```python
from build123d import *

# Parameters (mm, degrees)
SKETCH1_W           = 37.4
SKETCH1_H           = 57.2
BOSS_EXTRUDE1_DEPTH = 12.5
SHELL1_T            = -2
CUT_EXTRUDE1_DEPTH  = 70.475535262
SKETCH3_W           = 33
SKETCH3_H           = 8
BOSS_EXTRUDE2_DEPTH = 15
SKETCH4_W           = 5
SKETCH4_H           = 23
CUT_EXTRUDE2_DEPTH  = 82.955246934
FILLET2_R           = 1


with BuildPart() as part:
    # Sketch1 → Boss-Extrude1 (new body)
    with BuildSketch(Plane(origin=(0, 0, 0), x_dir=(0, 1, 0), z_dir=(0, 0, 1))):
        with Locations((-18.7, 28.6)):
            Rectangle(SKETCH1_W, SKETCH1_H)
    extrude(amount=BOSS_EXTRUDE1_DEPTH)

    # Shell1
    shell1_openings = [part.faces().sort_by_distance(p)[0] for p in [
        (0, -18.7, 6.25),
    ]]
    offset(amount=SHELL1_T, openings=shell1_openings, kind=Kind.INTERSECTION)

    # Sketch2 → Cut-Extrude1 (cut, through all)
    with BuildSketch(Plane.XY.offset(12.5)):
        with BuildLine():
            Line((-51.1, -37.4), (-51.1, -35.4))
            ThreePointArc((-51.1, -35.4), (-48.35, -32.65), (-45.6, -35.4))
            Line((-45.6, -35.4), (-45.6, -37.4))
            Line((-45.6, -37.4), (-51.1, -37.4))
        make_face()
        with BuildLine():
            Line((-51.1, 0), (-51.1, -2))
            ThreePointArc((-51.1, -2), (-48.35, -4.75), (-45.6, -2))
            Line((-45.6, -2), (-45.6, 0))
            Line((-45.6, 0), (-51.1, 0))
        make_face()
    extrude(amount=-CUT_EXTRUDE1_DEPTH, mode=Mode.SUBTRACT)

    # Sketch3 → Boss-Extrude2 (add)
    with BuildSketch(Plane(origin=(-57.2, 0, 0), x_dir=(0, -1, 0), z_dir=(-1, 0, 0))):
        with Locations((18.7, 6.25)):
            Rectangle(SKETCH3_W, SKETCH3_H)
    extrude(amount=BOSS_EXTRUDE2_DEPTH)

    # Sketch4 → Cut-Extrude2 (cut, through all)
    with BuildSketch(Plane(origin=(0, 0, 2.25), x_dir=(1, 0, 0), z_dir=(0, 0, -1))):
        with Locations((-64.7, 18.7)):
            Rectangle(SKETCH4_W, SKETCH4_H)
    extrude(amount=-CUT_EXTRUDE2_DEPTH, mode=Mode.SUBTRACT)

    # Fillet2
    fillet2_edges = [part.edges().sort_by_distance(p)[0] for p in [
        (-54.15, -37.4, 12.5),
        (-53.15, -35.4, 10.5),
        (-54.15, 0, 0),
        (-22.8, -37.4, 0),
        (-54.15, 0, 12.5),
        (-22.8, -37.4, 12.5),
        (-45.6, -37.4, 6.25),
        (-51.1, -37.4, 6.25),
        (-22.8, 0, 12.5),
        (-51.1, 0, 6.25),
        (-45.6, 0, 6.25),
        (-54.15, -37.4, 0),
        (-57.2, -18.7, 0),
        (-22.8, 0, 0),
        (-57.2, -35.2, 6.25),
        (-64.7, -35.2, 2.25),
        (-57.2, -18.7, 10.25),
        (-64.7, -35.2, 10.25),
        (-57.2, -2.2, 6.25),
        (-64.7, -2.2, 10.25),
        (-57.2, -18.7, 2.25),
        (-64.7, -2.2, 2.25),
        (-72.2, -35.2, 6.25),
        (-72.2, -18.7, 10.25),
        (-72.2, -2.2, 6.25),
        (-72.2, -18.7, 2.25),
        (-57.2, -37.4, 6.25),
        (-57.2, 0, 6.25),
        (-64.7, -7.2, 10.25),
        (-62.2, -7.2, 6.25),
        (-67.2, -18.7, 10.25),
        (-67.2, -7.2, 6.25),
        (-64.7, -30.2, 10.25),
        (-67.2, -30.2, 6.25),
        (-62.2, -18.7, 10.25),
        (-62.2, -30.2, 6.25),
        (-64.7, -7.2, 2.25),
        (-62.2, -18.7, 2.25),
        (-57.2, -18.7, 12.5),
        (-64.7, -30.2, 2.25),
        (-67.2, -18.7, 2.25),
    ]]
    fillet(fillet2_edges, radius=FILLET2_R)


solid = part.part
```
Verification items for the finished model (mm, model axes). A direction names the side the tool comes from. Coordinates: 2 decimals unless noted, no trailing zeros. Loops run counter-clockwise (first coordinate to the right, second up) from the corner with the lowest first, then second, coordinate; pieces in that order, holes last. Notation, with made-up numbers: (72.25, 25) -> (105.25, 25) arc R29 ccw to (105.25, 56) -> close; hole circle Ø1 at (-27.75, 5). An arc over 180 degrees is marked (long way). Answer in a Markdown table with one row per item. Add a question column.
1. Section check D-D, the plane z = 8. Give the number of separate pieces and of enclosed holes in the cut face, then the cut area to 3 significant figures.
2. Section check C-C, the plane x = -20. Enter the section's corners in (y, z).
3. Access from +Z, -Z, +X, -X, +Y, -Y to the whole of each face (thin tool, end or side, straight path). Record for faces 4 (the face through (-65, -35.2, 6)), 5 (the face through (-69, -18, 10.25)), 6 (the face through (-53, -2, 6)).
4. Material ranges on probe 1 along X at (y, z) = (-13.5, 8.75); probe 2 along Z at (x, y) = (-44, -35); probe 3 along Y at (x, z) = (-31, 9.25), recorded low to high. Write a range as [from, to].
5. Section check B-B, the plane y = -14. Enter the section's corners in (x, z), then the cut area to 3 significant figures.
6. Section check A-A, the plane x = -65. Enter the section's corners in (y, z).
7. Depth check by flat-ended pin: P1, Ø0.5, axis at y = -1.5, z = 8.5, coming from the -X side; P2, Ø5, axis at x = -64, z = 6, coming from the -Y side; P3, Ø1.5, axis at x = -65.5, z = 5, coming from the +Y side. Enter the tip coordinate at first touch or a pass-through.
8. Draft check along X on faces 1 (the face through (-55.2, -19, 6)), 2 (the face through (-65, -2.2, 6)), 3 (the face through (-48.41, -4.75, 11.51)). Enter one of: +X half, -X half, draft (parallel to the pull), parting line (faces both ways), or undercut.
Derived:
| question | item | result |
|---|---|---|
| 1 | separate pieces | 3 |
| 1 | enclosed holes | 1 |
| 1 | area | 653 mm² |
| 2 | outline | (-37.4, 1) arc R1 ccw to (-36.4, 0) -> (-1, 0) arc R1 ccw to (0, 1) -> (0, 11.5) arc R1 ccw to (-1, 12.5) -> (-36.4, 12.5) arc R1 ccw to (-37.4, 11.5) -> close; hole (-35.4, 2) -> (-2, 2) -> (-2, 10.5) -> (-35.4, 10.5) -> close |
| 3 | face 4 | +Z, -Z, -X, -Y |
| 3 | face 5 | +Z, -X, +Y, -Y |
| 3 | face 6 | +X |
| 4 | probe 1 | x = [-72.2, -67.2], [-62.2, -55.2] |
| 4 | probe 2 | z = [0, 2], [10.5, 12.5] |
| 4 | probe 3 | y = [-37.4, -35.4], [-2, 0] |
| 5 | outline | (-72.2, 3.25) arc R1 ccw to (-71.2, 2.25) -> (-68.2, 2.25) arc R1 ccw to (-67.2, 3.25) -> (-67.2, 9.25) arc R1 ccw to (-68.2, 10.25) -> (-71.2, 10.25) arc R1 ccw to (-72.2, 9.25) -> close; (-62.2, 3.25) arc R1 ccw to (-61.2, 2.25) -> (-58.2, 2.25) arc R1 cw to (-57.2, 1.25) -> (-57.2, 1) arc R1 ccw to (-56.2, 0) -> (0, 0) -> (0, 2) -> (-55.2, 2) -> (-55.2, 10.5) -> (0, 10.5) -> (0, 12.5) -> (-56.2, 12.5) arc R1 ccw to (-57.2, 11.5) -> (-57.2, 11.25) arc R1 cw to (-58.2, 10.25) -> (-61.2, 10.25) arc R1 ccw to (-62.2, 9.25) -> close |
| 5 | area | 325 mm² |
| 6 | outline | (-35.2, 3.25) arc R1 ccw to (-34.2, 2.25) -> (-31.2, 2.25) arc R1 ccw to (-30.2, 3.25) -> (-30.2, 9.25) arc R1 ccw to (-31.2, 10.25) -> (-34.2, 10.25) arc R1 ccw to (-35.2, 9.25) -> close; (-7.2, 3.25) arc R1 ccw to (-6.2, 2.25) -> (-3.2, 2.25) arc R1 ccw to (-2.2, 3.25) -> (-2.2, 9.25) arc R1 ccw to (-3.2, 10.25) -> (-6.2, 10.25) arc R1 ccw to (-7.2, 9.25) -> close |
| 7 | P1 | stops at x = -57.36 |
| 7 | P2 | stops at y = -35.2 |
| 7 | P3 | stops at y = -2.2 |
| 8 | face 1 | +X half |
| 8 | face 2 | draft |
| 8 | face 3 | undercut |
